Check sheet for the modelled part. Datum: model origin and axes. Units: mm. Face numbers are marked on the shaded views. A direction names the side the tool comes from. Coordinates: 2 decimals unless noted, no trailing zeros. Order: outer loops, then holes, each group sorted by start corner. A loop starts at its lowest first (then second) coordinate and runs counter-clockwise, first axis right, second up.
1. Cross-section at A-A (x = 7.45). Enter the section's corners in (y, z).
2. Cross-section at B-B (x = 5.5). Enter the section's corners in (y, z), then the cut area to 3 significant figures.
3. Cross-section at D-D (x = 9.75). Enter the section's corners in (y, z), then the cut area to 3 significant figures.
4. Set-up check for the marked faces 1, 2 and 3: record each of +Z, -Z, +X, -X, +Y, -Y from which the full face is reachable in a straight line by a thin tool's end or side.
5. Thickness scan on line 1 (X direction, y = 1.3, z = 1.82); line 2 (Z direction, x = 10.25, y = 3.7); line 3 (X direction, y = 2, z = 0.75). Record the ranges inside material, lowest first.
6. Draft check along Z on the marked faces 4, 5, 6 and 7. Enter one of: released by +Z, released by -Z, zero draft, split by the parting line, or undercut.
7. Cross-section at C-C (y = 0.8). Enter the section's corners in (x, z), then the cut area to 3 significant figures.
8. Gauge pin test, flat ends, axial feed: pin 1 Ø1 at (x, z) = (7, 3) entering from +Y; pin 2 Ø0.6 at (x, y) = (0.5, 4) entering from -Z. Record the tip position at first contact, or that the pin passes through.
```python
from build123d import *

# Parameters (mm, degrees)
SKETCH_1_W             = 12.4
SKETCH_1_H             = 5.9
EXTRUDE_1_DEPTH        = 4.9
CUT_EXTRUDE_1_DEPTH    = 4
SKETCH_4_W             = 1
SKETCH_4_H             = 1
SKETCH_4_W_2           = 2.2
SKETCH_4_H_2           = 0.1
CUT_EXTRUDE_2_DEPTH    = 15.580123456
SKETCH_5_W             = 0.7
SKETCH_5_H             = 1
CUT_EXTRUDE_3_DEPTH    = 2
CHAMFER_1_SIZE         = 1.2
SKETCH_6_R             = 0.35
CUT_EXTRUDE_4_DEPTH    = 15.539944979
PATTERN_LINEAR_1_COUNT = 4
PATTERN_LINEAR_1_PITCH = 2.5
CUT_EXTRUDE_5_REACH    = 16.205
SKETCH_7_W             = 0.7
SKETCH_7_H             = 1.8
EXTRUDE_2_DEPTH        = 3.5
PATTERN_LINEAR_2_COUNT = 3
PATTERN_LINEAR_2_PITCH = 2.5
CHAMFER_2_SIZE         = 0.3


with BuildPart() as part:
    # 스케치1 → 보스-돌출1 (new body)
    with BuildSketch(Plane.XY):
        with Locations((6.2, 2.95)):
            Rectangle(SKETCH_1_W, SKETCH_1_H)
    extrude(amount=EXTRUDE_1_DEPTH)

    # 스케치2 → 컷-돌출1 (cut)
    with BuildSketch(Plane(origin=(0, 5.9, 0), x_dir=(1, 0, 0), z_dir=(0, 1, 0))):
        Polygon((0.7, -1.5), (1.5, -0.7), (10.9, -0.7), (11.7, -1.5), (11.7, -4.2), (0.7, -4.2), align=None)
    extrude(amount=-CUT_EXTRUDE_1_DEPTH, mode=Mode.SUBTRACT)

    # 스케치4 → 컷-돌출2 (cut, through all)
    with BuildSketch(Plane(origin=(12.4, 0, 0), x_dir=(0, 0, -1), z_dir=(1, 0, 0))):
        with Locations((-4.4, 0.5)):
            Rectangle(SKETCH_4_W, SKETCH_4_H)
        with Locations((-1.95, 0.05)):
            Rectangle(SKETCH_4_W_2, SKETCH_4_H_2)
        Polygon((-3.7, 5.4), (-4.2, 5.9), (-2.2, 5.9), (-2.7, 5.4), (-2.7, 4.85), (-1.9, 4.85), (-1.9, 1.9), (-3.7, 1.9), align=None)
    extrude(amount=-CUT_EXTRUDE_2_DEPTH, mode=Mode.SUBTRACT)

    # 스케치5 → 컷-돌출3 (cut)
    with BuildSketch(Plane.XY.offset(3.9)):
        with Locations((0.35, 0.5)):
            Rectangle(SKETCH_5_W, SKETCH_5_H)
        with Locations((12.05, 0.5)):
            Rectangle(SKETCH_5_W, SKETCH_5_H)
    extrude(amount=-CUT_EXTRUDE_3_DEPTH, mode=Mode.SUBTRACT)

    # 모따기1
    chamfer_1_edges = [part.edges().sort_by_distance(p)[0] for p in [
        (0, 2.95, 0),
    ]]
    chamfer(chamfer_1_edges, length=CHAMFER_1_SIZE)

    # 스케치6 → 컷-돌출4 (cut, through all)
    with BuildSketch(Plane.XZ.offset(-0.1)):
        with Locations(Location((2.45, 1.82, 0), (0, 0, 270))):
            Circle(SKETCH_6_R)
    cut_extrude_4 = extrude(amount=-CUT_EXTRUDE_4_DEPTH, mode=Mode.SUBTRACT)

    # 선형 패턴1: 컷-돌출4 ×4
    with Locations(*[(i * PATTERN_LINEAR_1_PITCH, 0, 0) for i in range(1, PATTERN_LINEAR_1_COUNT)]):
        add(cut_extrude_4, mode=Mode.SUBTRACT)

    # 스케치7 → 컷-돌출5 (cut, up to next)
    with BuildSketch(Plane.XZ.offset(-1), mode=Mode.PRIVATE) as cut_extrude_5_sk1:
        with Locations((0.35, 2.8)):
            Rectangle(SKETCH_7_W, SKETCH_7_H)
    cut_extrude_5_tool1 = extrude(cut_extrude_5_sk1.sketch, amount=-CUT_EXTRUDE_5_REACH, mode=Mode.PRIVATE) & part.part
    # 스케치7 → 컷-돌출5 (cut, up to next)
    with BuildSketch(Plane.XZ.offset(-1), mode=Mode.PRIVATE) as cut_extrude_5_sk2:
        with Locations((12.05, 2.8)):
            Rectangle(SKETCH_7_W, SKETCH_7_H)
    cut_extrude_5_tool2 = extrude(cut_extrude_5_sk2.sketch, amount=-CUT_EXTRUDE_5_REACH, mode=Mode.PRIVATE) & part.part
    add(cut_extrude_5_tool1.solids().sort_by_distance((0.35, 1, 2.8))[0], mode=Mode.SUBTRACT)
    add(cut_extrude_5_tool2.solids().sort_by_distance((12.05, 1, 2.8))[0], mode=Mode.SUBTRACT)

    # 스케치8 → 보스-돌출2 (add)
    with BuildSketch(Plane(origin=(0, 1.9, 0), x_dir=(1, 0, 0), z_dir=(0, 1, 0))):
        Polygon((3.2, -0.7), (4.2, -0.7), (3.7, -1.2), align=None)
    extrude_2 = extrude(amount=EXTRUDE_2_DEPTH)

    # 선형 패턴2: 보스-돌출2 ×3
    with Locations(*[(i * PATTERN_LINEAR_2_PITCH, 0, 0) for i in range(1, PATTERN_LINEAR_2_COUNT)]):
        add(extrude_2)

    # 모따기2
    chamfer_2_edges = [part.edges().sort_by_distance(p)[0] for p in [
        (6.2, 5.9, 0.7),
        (6.2, 5.9, 4.2),
    ]]
    chamfer(chamfer_2_edges, length=CHAMFER_2_SIZE)


solid = part.part
```
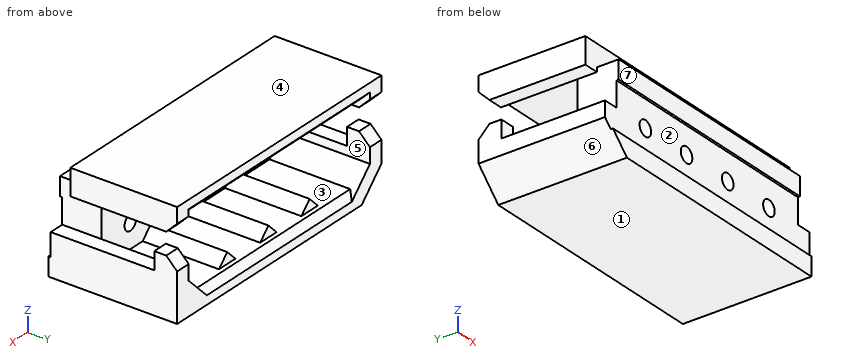
Data:
1. outline: (0, 0) - (5.9, 0) - (5.9, 0.4) - (5.6, 0.7) - (1.9, 0.7) - (1.9, 1.47) - (0.1, 1.47) - (0.1, 0.85) - (0, 0.85) - close; (0, 3.05) - (0.1, 3.05) - (0.1, 2.17) - (1.9, 2.17) - (1.9, 4.2) - (5.6, 4.2) - (5.9, 4.5) - (5.9, 4.9) - (1, 4.9) - (1, 3.9) - (0, 3.9) - close
2. outline: (0, 0) - (5.9, 0) - (5.9, 0.4) - (5.6, 0.7) - (1.9, 0.7) - (1.9, 4.2) - (5.6, 4.2) - (5.9, 4.5) - (5.9, 4.9) - (1, 4.9) - (1, 3.9) - (0, 3.9) - (0, 3.05) - (0.1, 3.05) - (0.1, 0.85) - (0, 0.85) - close
2. area: 13.6 mm2
3. outline: (0, 0) - (5.9, 0) - (5.9, 0.4) - (5.6, 0.7) - (1.9, 0.7) - (1.9, 1.53) - (0.1, 1.53) - (0.1, 0.85) - (0, 0.85) - close; (0, 3.05) - (0.1, 3.05) - (0.1, 2.11) - (1.9, 2.11) - (1.9, 4.2) - (5.6, 4.2) - (5.9, 4.5) - (5.9, 4.9) - (1, 4.9) - (1, 3.9) - (0, 3.9) - close
3. area: 12.6 mm2
4. face 1: -Z, +X, -X, +Y, -Y
4. face 2: +X, -X, -Y
4. face 3: +Y
5. line 1: x = 0 to 2.1, 2.8 to 4.6, 5.3 to 7.1, 7.8 to 9.6, 10.3 to 12.4
5. line 2: z = 0 to 0.7, 4.2 to 4.9
5. line 3: x = 0.45 to 1.45, 3.25 to 4.15, 5.75 to 6.65, 8.25 to 9.15, 10.95 to 12.4
6. face 4: released by +Z
6. face 5: undercut
6. face 6: released by -Z
6. face 7: zero draft
7. outline: (0, 1.2) - (1.2, 0) - (12.4, 0) - (12.4, 1.9) - (11.7, 1.9) - (11.7, 3.9) - (0.7, 3.9) - (0.7, 1.9) - (0, 1.9) - close; hole circle Ø0.7 at (2.45, 1.82); hole circle Ø0.7 at (4.95, 1.82); hole circle Ø0.7 at (7.45, 1.82); hole circle Ø0.7 at (9.95, 1.82)
7. area: 43.3 mm2
8. pin 1: stops at y = 1.9
8. pin 2: stops at z = 0.4
